from build123d import *

# Parameters (mm, degrees)
F1_W         = 203.2
F1_H         = 127
F2_DEPTH     = 76.2
F3_D         = 127
F3_DEPTH     = 76.2
F3_TIP       = 38.1546493083
F4_DEPTH     = 2.54
F5_T3_DEPTH  = 210.82
F5_T5_DEPTH  = 142.24
F5_T7_DEPTH  = 193.04
F5_T9_DEPTH  = 137.16
F5_T11_DEPTH = 119.38
F5_S15_W     = 5.08
F5_S15_H     = 5.08
F5_T16_DEPTH = 5.08
F5_S21_W     = 5.08
F5_S21_H     = 5.08
F5_T22_DEPTH = 5.08
F5_S27_W     = 5.08
F5_S27_H     = 5.08
F5_T28_DEPTH = 5.08
F5_S33_W     = 5.08
F5_S33_H     = 5.08
F5_T34_DEPTH = 5.08
F5_S39_W     = 5.08
F5_S39_H     = 5.08
F5_T40_DEPTH = 5.08
F5_S45_W     = 5.08
F5_S45_H     = 5.08
F5_T46_DEPTH = 5.08


# Not quite as in the source:
# - a fillet or chamfer that OpenCascade refuses, or shapes differently, is made with other operations: its cross-section is extruded or revolved along the edge and cut away or added


with BuildPart() as f2:
    # F1 (on Front) → F2 (new body, symmetric)
    with BuildSketch(Plane.XZ):
        with Locations((0, -63.5)):
            Rectangle(F1_W, F1_H)
    extrude(amount=F2_DEPTH, both=True)

    # F3
    with Locations(Plane.XY):
        with Locations((0, -3.3519673161)):
            Hole(F3_D / 2, depth=F3_DEPTH)
            with Locations((0, 0, -(F3_DEPTH + F3_TIP / 2))):  # 118° drill point
                Cone(0, F3_D / 2, F3_TIP, mode=Mode.SUBTRACT)

    # F4 (add): a face of the model
    f4_faces = [f2.faces().sort_by_distance(p)[0] for p in [
        (0, 0, -127),
    ]]
    extrude(f4_faces, amount=F4_DEPTH)

    # F5: fillet of radius 5.08 on 13 edges, made by hand

    # F5_s1 → F5_t2 (revolve)
    with BuildSketch(Plane.XZ.offset(3.3519673161)):
        with BuildLine():
            ThreePointArc((63.5, -73.3258742868), (62.8414069354, -75.8273859721), (61.0363934205, -77.6802841744))
            Line((61.0363934205, -77.6802841744), (63.5, -76.2))
            Line((63.5, -76.2), (63.5, -73.3258742868))
        make_face()
    revolve(axis=Axis((0, -3.3519673161, -76.2), (0, 0, 1)))

    # F5_s4 → F5_t3 (cut)
    with BuildSketch(Plane.YZ.offset(-114.3)):
        with BuildLine():
            ThreePointArc((71.12, 0), (74.7121024484, -1.4878975516), (76.2, -5.08))
            Line((76.2, -5.08), (76.2, 0))
            Line((76.2, 0), (71.12, 0))
        make_face()
        with BuildLine():
            ThreePointArc((-71.12, 0), (-74.7121024484, -1.4878975516), (-76.2, -5.08))
            Line((-76.2, -5.08), (-76.2, 0))
            Line((-76.2, 0), (-71.12, 0))
        make_face()
    extrude(amount=F5_T3_DEPTH, mode=Mode.SUBTRACT)

    # F5_s6 → F5_t5 (cut)
    with BuildSketch(Plane.XZ.offset(-71.12)):
        with BuildLine():
            ThreePointArc((101.6, -5.08), (100.1121024484, -1.4878975516), (96.52, 0))
            Line((96.52, 0), (101.6, 0))
            Line((101.6, 0), (101.6, -5.08))
        make_face()
        with BuildLine():
            ThreePointArc((101.6, -124.46), (100.1121024484, -128.0521024484), (96.52, -129.54))
            Line((96.52, -129.54), (101.6, -129.54))
            Line((101.6, -129.54), (101.6, -124.46))
        make_face()
        with BuildLine():
            ThreePointArc((-96.52, -129.54), (-100.1121024484, -128.0521024484), (-101.6, -124.46))
            Line((-101.6, -124.46), (-101.6, -129.54))
            Line((-101.6, -129.54), (-96.52, -129.54))
        make_face()
    extrude(amount=F5_T5_DEPTH, mode=Mode.SUBTRACT)

    # F5_s8 → F5_t7 (cut)
    with BuildSketch(Plane.YZ.offset(-96.52)):
        with BuildLine():
            ThreePointArc((-76.2, -124.46), (-74.7121024484, -128.0521024484), (-71.12, -129.54))
            Line((-71.12, -129.54), (-76.2, -129.54))
            Line((-76.2, -129.54), (-76.2, -124.46))
        make_face()
        with BuildLine():
            ThreePointArc((71.12, -129.54), (74.7121024484, -128.0521024484), (76.2, -124.46))
            Line((76.2, -124.46), (76.2, -129.54))
            Line((76.2, -129.54), (71.12, -129.54))
        make_face()
    extrude(amount=F5_T7_DEPTH, mode=Mode.SUBTRACT)

    # F5_s10 → F5_t9 (cut)
    with BuildSketch(Plane.XY.offset(-124.46)):
        with BuildLine():
            ThreePointArc((-96.52, -76.2), (-100.1121024484, -74.7121024484), (-101.6, -71.12))
            Line((-101.6, -71.12), (-101.6, -76.2))
            Line((-101.6, -76.2), (-96.52, -76.2))
        make_face()
        with BuildLine():
            ThreePointArc((-96.52, 76.2), (-100.1121024484, 74.7121024484), (-101.6, 71.12))
            Line((-101.6, 71.12), (-101.6, 76.2))
            Line((-101.6, 76.2), (-96.52, 76.2))
        make_face()
    extrude(amount=F5_T9_DEPTH, mode=Mode.SUBTRACT)

    # F5_s12 → F5_t11 (cut)
    with BuildSketch(Plane.XY.offset(-124.46)):
        with BuildLine():
            ThreePointArc((101.6, -71.12), (100.1121024484, -74.7121024484), (96.52, -76.2))
            Line((96.52, -76.2), (101.6, -76.2))
            Line((101.6, -76.2), (101.6, -71.12))
        make_face()
        with BuildLine():
            ThreePointArc((101.6, 71.12), (100.1121024484, 74.7121024484), (96.52, 76.2))
            Line((96.52, 76.2), (101.6, 76.2))
            Line((101.6, 76.2), (101.6, 71.12))
        make_face()
    extrude(amount=F5_T11_DEPTH, mode=Mode.SUBTRACT)


with BuildPart() as f5_tool14:
    # F5_s15 → F5_t16 (new body)
    with BuildSketch(Plane.YZ.offset(96.52)):
        with Locations((73.66, -2.54)):
            Rectangle(F5_S15_W, F5_S15_H)
    extrude(amount=F5_T16_DEPTH)

    # F5_s17 → F5_t18 (revolve, cut)
    with BuildSketch(Plane(origin=(96.52, 71.12, -5.08), x_dir=(0, -0.7071067812, -0.7071067812), z_dir=(0, -0.7071067812, 0.7071067812))):
        with BuildLine():
            ThreePointArc((0, -5.08), (5.08, 0), (0, 5.08))
            Line((0, 5.08), (0, -5.08))
        make_face()
    revolve(axis=Axis((96.52, 71.12, -5.08), (1, 0, 0)), mode=Mode.SUBTRACT)


with BuildPart() as f2_1:
    add(f2.part)

    # F5_t13: cut F5_tool14
    add(f5_tool14.part, mode=Mode.SUBTRACT)


with BuildPart() as f5_tool20:
    # F5_s21 → F5_t22 (new body)
    with BuildSketch(Plane.YZ.offset(96.52)):
        with Locations((-73.66, -2.54)):
            Rectangle(F5_S21_W, F5_S21_H)
    extrude(amount=F5_T22_DEPTH)

    # F5_s23 → F5_t24 (revolve, cut)
    with BuildSketch(Plane(origin=(96.52, -71.12, -5.08), x_dir=(0, 0.7071067812, -0.7071067812), z_dir=(0, -0.7071067812, -0.7071067812))):
        with BuildLine():
            ThreePointArc((0, -5.08), (5.08, 0), (0, 5.08))
            Line((0, 5.08), (0, -5.08))
        make_face()
    revolve(axis=Axis((96.52, -71.12, -5.08), (1, 0, 0)), mode=Mode.SUBTRACT)


with BuildPart() as f2_2:
    add(f2_1.part)

    # F5_t19: cut F5_tool20
    add(f5_tool20.part, mode=Mode.SUBTRACT)


with BuildPart() as f5_tool26:
    # F5_s27 → F5_t28 (new body)
    with BuildSketch(Plane.YZ.offset(96.52)):
        with Locations((-73.66, -127)):
            Rectangle(F5_S27_W, F5_S27_H)
    extrude(amount=F5_T28_DEPTH)

    # F5_s29 → F5_t30 (revolve, cut)
    with BuildSketch(Plane(origin=(96.52, -71.12, -124.46), x_dir=(0, 0.7071067812, 0.7071067812), z_dir=(0, 0.7071067812, -0.7071067812))):
        with BuildLine():
            ThreePointArc((0, -5.08), (5.08, 0), (0, 5.08))
            Line((0, 5.08), (0, -5.08))
        make_face()
    revolve(axis=Axis((96.52, -71.12, -124.46), (1, 0, 0)), mode=Mode.SUBTRACT)


with BuildPart() as f2_3:
    add(f2_2.part)

    # F5_t25: cut F5_tool26
    add(f5_tool26.part, mode=Mode.SUBTRACT)


with BuildPart() as f5_tool32:
    # F5_s33 → F5_t34 (new body)
    with BuildSketch(Plane.YZ.offset(96.52)):
        with Locations((73.66, -127)):
            Rectangle(F5_S33_W, F5_S33_H)
    extrude(amount=F5_T34_DEPTH)

    # F5_s35 → F5_t36 (revolve, cut)
    with BuildSketch(Plane(origin=(96.52, 71.12, -124.46), x_dir=(0, -0.7071067812, 0.7071067812), z_dir=(0, 0.7071067812, 0.7071067812))):
        with BuildLine():
            ThreePointArc((0, -5.08), (5.08, 0), (0, 5.08))
            Line((0, 5.08), (0, -5.08))
        make_face()
    revolve(axis=Axis((96.52, 71.12, -124.46), (1, 0, 0)), mode=Mode.SUBTRACT)


with BuildPart() as f2_4:
    add(f2_3.part)

    # F5_t31: cut F5_tool32
    add(f5_tool32.part, mode=Mode.SUBTRACT)


with BuildPart() as f5_tool38:
    # F5_s39 → F5_t40 (new body)
    with BuildSketch(Plane.XZ.offset(71.12)):
        with Locations((-99.06, -127)):
            Rectangle(F5_S39_W, F5_S39_H)
    extrude(amount=F5_T40_DEPTH)

    # F5_s41 → F5_t42 (revolve, cut)
    with BuildSketch(Plane(origin=(-96.52, -71.12, -124.46), x_dir=(0.7071067812, 0, 0.7071067812), z_dir=(0.7071067812, 0, -0.7071067812))):
        with BuildLine():
            ThreePointArc((0, -5.08), (5.08, 0), (0, 5.08))
            Line((0, 5.08), (0, -5.08))
        make_face()
    revolve(axis=Axis((-96.52, -71.12, -124.46), (0, -1, 0)), mode=Mode.SUBTRACT)


with BuildPart() as f2_5:
    add(f2_4.part)

    # F5_t37: cut F5_tool38
    add(f5_tool38.part, mode=Mode.SUBTRACT)


with BuildPart() as f5_tool44:
    # F5_s45 → F5_t46 (new body)
    with BuildSketch(Plane.XY.offset(-124.46)):
        with Locations((-99.06, 73.66)):
            Rectangle(F5_S45_W, F5_S45_H)
    extrude(amount=-F5_T46_DEPTH)

    # F5_s47 → F5_t48 (revolve, cut)
    with BuildSketch(Plane(origin=(-96.52, 71.12, -124.46), x_dir=(0.7071067812, -0.7071067812, 0), z_dir=(0.7071067812, 0.7071067812, 0))):
        with BuildLine():
            ThreePointArc((0, -5.08), (5.08, 0), (0, 5.08))
            Line((0, 5.08), (0, -5.08))
        make_face()
    revolve(axis=Axis((-96.52, 71.12, -124.46), (0, 0, -1)), mode=Mode.SUBTRACT)


with BuildPart() as f2_6:
    add(f2_5.part)

    # F5_t43: cut F5_tool44
    add(f5_tool44.part, mode=Mode.SUBTRACT)

    # F5_s49 → F5_t50 (revolve, cut)
    with BuildSketch(Plane.XZ.offset(3.3519673161)):
        with BuildLine():
            ThreePointArc((68.58, 0), (64.9878975516, -1.4878975516), (63.5, -5.08))
            Line((63.5, -5.08), (63.5, 0))
            Line((63.5, 0), (68.58, 0))
        make_face()
    revolve(axis=Axis((0, -3.3519673161, 0), (0, 0, 1)), mode=Mode.SUBTRACT)


solid = f2_6.part
The listing builds one solid part. Answer for the finished solid, in the listing's coordinates (mm). Give positions to 0.01 mm unless a question says otherwise; leave off trailing zeros. Write each loop counter-clockwise with the first axis right and the second up, starting at its lowest first coordinate (ties: lowest second). Pieces come first, ordered by that corner, then holes.
1) For a pull along Y with two mould halves and no side action, classify faces 1 (the face through (-1.351, -74.751, -128.012)), 2 (the face through (-60.57, 15.72, -39.68)), 3 (the face through (-3.927, 74.672, -1.449)) as pulls with the +Y half, pulls with the -Y half, needs draft (parallel to the pull), parting line crosses it, or undercut.
2) Section B-B (z = -19) is taken. Write down the section's boundary in (x, y), and give its area (3 significant figures).
3) Section A-A (z = -83) is taken. Write down the section's boundary in (x, y), and give its area (3 significant figures).
4) Find the intervals of material crossed by L1, parallel to X at y = -4, z = -57; L2, parallel to Y at x = 0, z = -24; L3, parallel to X at y = -23.5, z = -91, in increasing order.
5) Given P1, Ø3, axis at x = 53.5, y = -41, coming from the +Z side; P2, Ø6, axis at x = -37, y = 34, coming from the +Z side, each flat-ended and moving along its own axis, determine where each tip first touches the part or whether it passes through.
Response:
1. face 1: pulls with the -Y half
1. face 2: undercut
1. face 3: pulls with the +Y half
2. outline: (-101.6, -71.12) arc R5.08 ccw to (-96.52, -76.2) - (96.52, -76.2) arc R5.08 ccw to (101.6, -71.12) - (101.6, 71.12) arc R5.08 ccw to (96.52, 76.2) - (-96.52, 76.2) arc R5.08 ccw to (-101.6, 71.12) - close; hole circle Ø127 at (0, -3.35)
2. area: 18,300 mm2
3. outline: (-101.6, -71.12) arc R5.08 ccw to (-96.52, -76.2) - (96.52, -76.2) arc R5.08 ccw to (101.6, -71.12) - (101.6, 71.12) arc R5.08 ccw to (96.52, 76.2) - (-96.52, 76.2) arc R5.08 ccw to (-101.6, 71.12) - close; hole circle Ø104.37 at (0, -3.35)
3. area: 22,400 mm2
4. L1: x = -101.6 to -63.5, 63.5 to 101.6
4. L2: y = -76.2 to -66.85, 60.15 to 76.2
4. L3: x = -101.6 to -33.24, 33.24 to 101.6
5. P1: stops at z = -0.28
5. P2: stops at z = -80.96
